Part model, mm, in its own coordinate system. A direction names the side the tool comes from. Coordinates: 2 decimals unless noted, no trailing zeros. Loops run counter-clockwise (first coordinate to the right, second up) from the corner with the lowest first, then second, coordinate; pieces in that order, holes last. Notation, with made-up numbers: (88.25, 78) - (103.25, 78) arc R20 ccw to (103.25, 117) - close; hole circle Ø2 at (-26.75, -37.75). An arc over 180 degrees is marked (long way). Answer as CSV lines item,"result".
from build123d import *

# Parameters (mm, degrees)
SKETCH1_W               = 27
SKETCH1_H               = 22
SKETCH1_R               = 1.5
BOSS_EXTRUDE1_DEPTH     = 3
SKETCH2_W               = 5
SKETCH2_H               = 18
BOSS_EXTRUDE2_DEPTH     = 23
CUT_EXTRUDE1_DEPTH      = 33.449961479
CUT_EXTRUDE1_DEPTH_BACK = 33.449961479
SKETCH3_R               = 4
CUT_EXTRUDE2_DEPTH      = 33.449961479
CUT_EXTRUDE2_DEPTH_BACK = 33.449961479
SKETCH4_W               = 9.515030356
SKETCH4_H               = 1.5
FILLET1_R               = 3
CUT_EXTRUDE3_DEPTH      = 37.636730203
CUT_EXTRUDE3_DEPTH_BACK = 37.636730203
SKETCH5_R               = 1.5
FILLET2_R               = 2
FILLET3_R               = 3


with BuildPart() as part:
    # Sketch1 → Boss-Extrude1 (new body)
    with BuildSketch(Plane.XY):
        Rectangle(SKETCH1_W, SKETCH1_H)
        with Locations((-10.5, -8.5)):
            Circle(SKETCH1_R, mode=Mode.SUBTRACT)
        with Locations((-10.5, 8.5)):
            Circle(SKETCH1_R, mode=Mode.SUBTRACT)
        with Locations((10.5, 8.5)):
            Circle(SKETCH1_R, mode=Mode.SUBTRACT)
        with Locations((10.5, -8.5)):
            Circle(SKETCH1_R, mode=Mode.SUBTRACT)
    extrude(amount=BOSS_EXTRUDE1_DEPTH)

    # Sketch2 → Boss-Extrude2 (add)
    with BuildSketch(Plane.XY.offset(3)):
        Rectangle(SKETCH2_W, SKETCH2_H)
    extrude(amount=BOSS_EXTRUDE2_DEPTH)

    # Sketch3 → Cut-Extrude1 (cut, two sides: drawn at the far end of the back side and taken through both)
    with BuildSketch(Plane(origin=(2.5, 0, 0), x_dir=(0, 0, -1), z_dir=(1, 0, 0)).offset(-CUT_EXTRUDE1_DEPTH_BACK)):
        with Locations(Location((-18, 0, 0), (0, 0, 180))):
            Circle(SKETCH3_R)
    extrude(amount=CUT_EXTRUDE1_DEPTH + CUT_EXTRUDE1_DEPTH_BACK, mode=Mode.SUBTRACT)

    # Sketch4 → Cut-Extrude2 (cut, two sides: drawn at the far end of the back side and taken through both)
    with BuildSketch(Plane(origin=(2.5, 0, 0), x_dir=(0, 0, -1), z_dir=(1, 0, 0)).offset(-CUT_EXTRUDE2_DEPTH_BACK)):
        with Locations((-21.491106051, 0)):
            Rectangle(SKETCH4_W, SKETCH4_H)
    extrude(amount=CUT_EXTRUDE2_DEPTH + CUT_EXTRUDE2_DEPTH_BACK, mode=Mode.SUBTRACT)

    # Fillet1
    fillet1_edges = [part.edges().sort_by_distance(p)[0] for p in [
        (-2.5, 0, 3),
        (2.5, 0, 3),
    ]]
    fillet(fillet1_edges, radius=FILLET1_R)

    # Sketch5 → Cut-Extrude3 (cut, two sides: drawn at the far end of the back side and taken through both)
    with BuildSketch(Plane(origin=(0, 11, 0), x_dir=(1, 0, 0), z_dir=(0, 1, 0)).offset(-CUT_EXTRUDE3_DEPTH_BACK)):
        with Locations(Location((0, -18, 0), (0, 0, 270))):
            Circle(SKETCH5_R)
    extrude(amount=CUT_EXTRUDE3_DEPTH + CUT_EXTRUDE3_DEPTH_BACK, mode=Mode.SUBTRACT)

    # Fillet2
    fillet2_edges = [part.edges().sort_by_distance(p)[0] for p in [
        (0, -9, 3),
        (0, 9, 3),
    ]]
    fillet(fillet2_edges, radius=FILLET2_R - 0.0001)  # a hair under: the kernel refuses the full size

    # Fillet3
    fillet3_edges = [part.edges().sort_by_distance(p)[0] for p in [
        (0, -9, 26),
        (0, 9, 26),
    ]]
    fillet(fillet3_edges, radius=FILLET3_R)


solid = part.part
Q1. Saw through at A-A (z = 18). Give the cut face in (x, y), then the cut area to 3 significant figures.
Results:
outline,"(-2.5, -9) - (-1.5, -9) - (-1.5, -4) - (-2.5, -4) - close; (-2.5, 4) - (-1.5, 4) - (-1.5, 9) - (-2.5, 9) - close; (1.5, -9) - (2.5, -9) - (2.5, -4) - (1.5, -4) - close; (1.5, 4) - (2.5, 4) - (2.5, 9) - (1.5, 9) - close"
area,"20.0 mm^2"
Q2. Wall check: L1, parallel to Y at x = 10.5, z = 1.95; L2, parallel to Z at x = 11.25, y = -4.5; L3, parallel to X at y = 8.5, z = 6.25. Give the ranges that are in metal, low to high.
Results:
L1,"y = -11 to -10, -7 to 7, 10 to 11"
L2,"z = 0 to 3"
L3,"x = -2.5 to 2.5"
Q3. Two-plate mould, pull along Y, no slides. Class faces 4 (the face through (-11.7, -9.4, 1.5)), 5 (the face through (0, 11, 1)), 6 (the face through (0.04, -8.1, 25.14)): released by +Y, released by -Y, zero draft, split by the parting line, or undercut.
Results:
face 4,"undercut"
face 5,"released by +Y"
face 6,"released by -Y"
Q4. Flat gauge pins, fed straight in: pin 1 (10.5 mm diameter, centred on y = 0, z = 18, fed in from -X); pin 2 (5 mm diameter, centred on x = -10.5, y = 8.5, fed in from +Z); pin 3 (9 mm diameter, centred on y = 3, z = 12.5, fed in from +X); pin 4 (1 mm diameter, centred on x = 2.5, y = -6, fed in from -Z). Where does each tip first touch, or does it go through?
Results:
pin 1,"stops at x = -2.5"
pin 2,"stops at z = 3"
pin 3,"stops at x = 2.5"
pin 4,"stops at z = 0"
Q5. Which spindle directions (+Z, -Z, +X, -X, +Y, -Y) get a long thin tool onto all of the face, cutting with end or side? Do faces 1 (the face through (6, 0, 3)), 2 (the face through (0, -9, 14)), 3 (the face through (0, 0.75, 24)). Say none if no direction does.
Results:
face 1,"+Z, +Y, -Y"
face 2,"+Z, +X, -X, -Y"
face 3,"+Z, +X, -X"
Q6. Saw through at D-D (y = -7.5). Give the cut face in (x, z).
Results:
outline,"(-13.5, 0) - (-11.62, 0) - (-11.62, 3) - (-13.5, 3) - close; (-9.38, 0) - (9.38, 0) - (9.38, 3) - (5.5, 3) arc R3 cw to (2.5, 6) - (2.5, 25.6) - (-2.5, 25.6) - (-2.5, 6) arc R3 cw to (-5.5, 3) - (-9.38, 3) - close; (11.62, 0) - (13.5, 0) - (13.5, 3) - (11.62, 3) - close; hole circle Ø3 at (0, 18)"
Q7. Saw through at C-C (z = 22.5). Give the cut face in (x, y), then the cut area to 3 significant figures.
Results:
outline,"(-2.5, -9) - (2.5, -9) - (2.5, -0.75) - (-2.5, -0.75) - close; (-2.5, 0.75) - (2.5, 0.75) - (2.5, 9) - (-2.5, 9) - close"
area,"82.5 mm^2"
Q8. Saw through at B-B (x = 10.5). Give the cut face in (y, z).
Results:
outline,"(-11, 0) - (-10, 0) - (-10, 3) - (-11, 3) - close; (-7, 0) - (7, 0) - (7, 3) - (-7, 3) - close; (10, 0) - (11, 0) - (11, 3) - (10, 3) - close"
